Verification items for the finished model (mm, model axes). Coordinates: 2 decimals unless noted, no trailing zeros. Loops run counter-clockwise (first coordinate to the right, second up) from the corner with the lowest first, then second, coordinate; pieces in that order, holes last. Notation, with made-up numbers: (-39, 45) - (-24, 45) arc R30 ccw to (-24, 81) - close; hole circle Ø4 at (-25, 68.25). An arc over 180 degrees is marked (long way). One line per item, written item: value. Start each with the question number.
(1) Section check B-B (z = 13.75). Record the boundary of the cut face in (x, y), plus the area to 3 significant figures.
(2) Section check C-C (z = 1.5). Record the boundary of the cut face in (x, y).
(3) Section check A-A (x = 29.5). Record the boundary of the cut face in (y, z), plus the area to 3 significant figures.
(4) Thickness scan on probe 1 along Y at (x, z) = (-5, 2.5); probe 2 along Z at (x, y) = (-11.5, 8); probe 3 along Y at (x, z) = (8, 4.25). Record the ranges inside material, lowest first. Write a range as [from, to].
```python
from build123d import *

# Parameters (mm, degrees)
F0_W     = 64.712018
F0_H     = 41.106358
F1_DEPTH = 25.4
F2_SIZE  = 5.08
F3_SIZE  = 5.08


with BuildPart() as f1:
    # F0 (on Top) → F1 (new body)
    with BuildSketch(Plane.XY):
        with Locations((5.08742, -7.732876)):
            Rectangle(F0_W, F0_H)
    extrude(amount=F1_DEPTH)

    # F2
    f2_edges = [f1.edges().sort_by_distance(p)[0] for p in [
        (5.08742, 12.820303, 25.4),
        (37.443429, -7.732876, 0),
        (37.443429, 12.820303, 12.7),
        (-27.268589, 12.820303, 12.7),
        (-27.268589, -7.732876, 25.4),
        (-27.268589, -7.732876, 0),
        (-27.268589, -28.286055, 12.7),
        (5.08742, -28.286055, 0),
        (5.08742, -28.286055, 25.4),
        (37.443429, -28.286055, 12.7),
        (37.443429, -7.732876, 25.4),
    ]]
    chamfer(f2_edges, length=F2_SIZE)

    # F3
    f3_edges = [f1.edges().sort_by_distance(p)[0] for p in [
        (5.08742, 12.820303, 0),
    ]]
    chamfer(f3_edges, length=F3_SIZE)


solid = f1.part
```
Responses:
1. outline: (-27.27, -23.21) - (-22.19, -28.29) - (32.36, -28.29) - (37.44, -23.21) - (37.44, 7.74) - (32.36, 12.82) - (-22.19, 12.82) - (-27.27, 7.74) - close
1. area: 2,610 mm²
2. outline: (-23.69, -23.21) - (-22.19, -24.71) - (32.36, -24.71) - (33.86, -23.21) - (33.86, 9.24) - (-23.69, 9.24) - close
3. outline: (-28.29, 5.08) - (-23.21, 0) - (7.74, 0) - (12.82, 5.08) - (12.82, 20.32) - (7.74, 25.4) - (-23.21, 25.4) - (-28.29, 20.32) - close
3. area: 992 mm²
4. probe 1: y = [-25.71, 10.24]
4. probe 2: z = [0.26, 25.14]
4. probe 3: y = [-27.46, 11.99]
